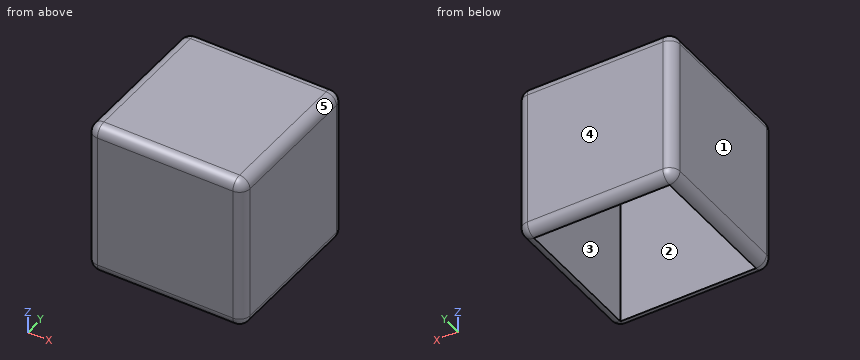
from build123d import *

# Parameters (mm, degrees)
F0_W     = 76.2
F0_H     = 76.2
F1_DEPTH = 76.2
F2_T     = -5.08
F3_R     = 5.07999


# Not quite as in the source:
# - a fillet or chamfer is up to 0.001 mm smaller than in the source, because OpenCascade refuses the exact size


with BuildPart() as f1:
    # F0 (on Front) → F1 (new body)
    with BuildSketch(Plane.XZ):
        with Locations((38.1, 38.1)):
            Rectangle(F0_W, F0_H)
    extrude(amount=F1_DEPTH)

    # F2
    f2_openings = [f1.faces().sort_by_distance(p)[0] for p in [
        (38.1, -38.1, 0),
    ]]
    offset(amount=F2_T, openings=f2_openings)

    # F3 (radius 5.08 in the source; OpenCascade refuses exactly that, so slightly less here)
    f3_edges = [f1.edges().sort_by_distance(p)[0] for p in [
        (76.2, -38.1, 76.2),
        (0, -38.1, 76.2),
        (38.1, 0, 76.2),
        (38.1, -76.2, 76.2),
        (76.2, -38.1, 0),
        (76.2, 0, 38.1),
        (76.2, -76.2, 38.1),
        (0, 0, 38.1),
        (0, -76.2, 38.1),
        (38.1, -76.2, 0),
        (0, -38.1, 0),
        (38.1, 0, 0),
    ]]
    fillet(f3_edges, radius=F3_R)


solid = f1.part
Read the model definition and answer for the solid it produces. Units are mm, in the model's axes. Face numbers are marked on the shaded views. A direction names the side the tool comes from. Coordinates: 2 decimals unless noted, no trailing zeros. Loops run counter-clockwise (first coordinate to the right, second up) from the corner with the lowest first, then second, coordinate; pieces in that order, holes last. Notation, with made-up numbers: (-12, -15) -> (38, -15) arc R33 cw to (38, 14) -> close; hole circle Ø11 at (39, 4.25). An arc over 180 degrees is marked (long way). Answer in a Markdown table with one row per item.
Item 1: For a pull along Y with two mould halves and no side action, classify the marked faces 3, 4 and 5 as released by +Y, released by -Y, zero draft, split by the parting line, or undercut.
Returned:
| item | result |
|---|---|
| face 3 | undercut |
| face 4 | released by +Y |
| face 5 | zero draft |
Item 2: For the marked faces 1 and 2, determine the directions among +Z, -Z, +X, -X, +Y, -Y from which every point of the face is accessible in a straight line to the end or side of a thin tool.
Returned:
| item | result |
|---|---|
| face 1 | +Z, -Z, -X, +Y, -Y |
| face 2 | -Z |
Item 3: A cutting plane is placed at B-B on z = 57. Determine the outline of the cut face in (x, y).
Returned:
| item | result |
|---|---|
| outline | (0, -71.12) arc R5.08 ccw to (5.08, -76.2) -> (71.12, -76.2) arc R5.08 ccw to (76.2, -71.12) -> (76.2, -5.08) arc R5.08 ccw to (71.12, 0) -> (5.08, 0) arc R5.08 ccw to (0, -5.08) -> close; hole (5.08, -71.12) -> (71.12, -71.12) -> (71.12, -5.08) -> (5.08, -5.08) -> close |
Item 4: This flat-tipped pin is pushed along its axis until it touches: P1, Ø2, axis at x = 67.5, y = -59, coming from the -Z side. Where does it stop, or does it pass through?
Returned:
| item | result |
|---|---|
| P1 | stops at z = 71.12 |
Item 5: Straight lines are drawn through the part: line 1 along X through (y, z) = (-29, 11.5); line 2 along Y through (x, z) = (70.5, 14); line 3 along Z through (x, y) = (43, -7.5). For each, find the intervals that lie inside material, in ascending order. Write a range as [from, to].
Returned:
| item | result |
|---|---|
| line 1 | x = [0, 5.08], [71.12, 76.2] |
| line 2 | y = [-76.2, -71.12], [-5.08, 0] |
| line 3 | z = [71.12, 76.2] |
